Read the model definition and answer for the solid it produces. Units are mm, in the model's axes. A direction names the side the tool comes from. Coordinates: 2 decimals unless noted, no trailing zeros. Write each loop counter-clockwise with the first axis right and the second up, starting at its lowest first coordinate (ties: lowest second). Pieces come first, ordered by that corner, then holes.
1) The part is cut by section C-C (x = -50). Determine the outline of the cut face in (y, z).
2) Each of these flat-tipped pins is pushed along its axis until it touches: pin 1 Ø1 at (y, z) = (-2, 3) entering from +X; pin 2 Ø4 at (x, y) = (-30.5, 26) entering from +Z; pin 3 Ø22.5 at (x, y) = (-50, 0) entering from +Z; pin 4 Ø2 at (x, y) = (-2.5, 16) entering from +Z. Where does it stop, or does it pass through?
3) The part is cut by section D-D (x = -27). Determine the outline of the cut face in (y, z).
4) Find the intervals of material crossed by line 1 (X direction, y = -19, z = 1); line 2 (Y direction, x = -50, z = 9.5); line 3 (Y direction, x = 0, z = 3.1), in increasing order.
5) Which of the six approach directions +Z, -Z, +X, -X, +Y, -Y give full straight-line access (tool end or side, diameter ignored) to faces 1 (the face through (5.2, -1, 3)), 2 (the face through (27.09, 0.37, 8.7)), 3 (the face through (-50.1, 14.4, 8))?
6) The part is cut by section B-B (y = 0). Give the number of separate pieces and of enclosed holes in the cut face, then the cut area to 3 significant figures.
7) The part is cut by section A-A (x = 1.5). Determine the outline of the cut face in (y, z), then the cut area to 3 significant figures.
from build123d import *
from OCP.BRepFilletAPI import BRepFilletAPI_MakeChamfer

# Parameters (mm, degrees)
SKETCH1_R               = 3
SKETCH1_R_2             = 16.15
BOSS_EXTRUDE1_DEPTH     = 12
CUT_EXTRUDE1_DEPTH      = 82.610354735
CUT_EXTRUDE1_DEPTH_BACK = 82.610354735
CUT_EXTRUDE2_DEPTH      = 81.984566431
CUT_EXTRUDE2_DEPTH_BACK = 81.984566431
CUT_EXTRUDE3_DEPTH      = 81.984566431
CUT_EXTRUDE3_DEPTH_BACK = 81.984566431
FILLET1_R               = 1.5
SKETCH5_R               = 18.073165259
SKETCH5_R_2             = 14
BOSS_EXTRUDE2_DEPTH     = 1.5
FILLET2_R               = 5
CHAMFER1_SIZE           = 2
CHAMFER1_SIZE2          = 1.908627476
SKETCH7_R               = 18.5
CUT_EXTRUDE4_DEPTH      = 81.984566431
CHAMFER2_SIZE           = 2
CHAMFER3_SIZE           = 1.5


with BuildPart() as part:
    # Sketch1 → Boss-Extrude1 (new body)
    with BuildSketch(Plane.XY):
        Polygon((-72, 16), (-72, -16), (-55.5, -26), (-16.944232072, -28.942026003), (-8.689847933, -35.598787405), (0, -36.5), (8.689847933, -35.598787405), (16.944232072, -28.942026003), (55.5, -26), (72, -16), (72, 16), (55.5, 26), (16.944232072, 28.942026003), (8.689847933, 35.598787405), (0, 36.5), (-8.689847933, 35.598787405), (-16.944232072, 28.942026003), (-55.5, 26), align=None)
        with Locations((0, 30)):
            Circle(SKETCH1_R, mode=Mode.SUBTRACT)
        with Locations((-50, 0)):
            Circle(SKETCH1_R_2, mode=Mode.SUBTRACT)
        with Locations(Location((0, -30, 0), (0, 0, 180))):
            Circle(SKETCH1_R, mode=Mode.SUBTRACT)
        with Locations(Location((50, 0, 0), (0, 0, 180))):
            Circle(SKETCH1_R_2, mode=Mode.SUBTRACT)
    extrude(amount=BOSS_EXTRUDE1_DEPTH)

    # Sketch2 → Cut-Extrude1 (cut, two sides)
    with BuildSketch(Plane(origin=(0, 0, 0), x_dir=(1, 0, 0), z_dir=(0, 1, 0))) as cut_extrude1_sk:
        Polygon((-31, -12), (-23.3, -5.5), (4.394576276, -5.5), (23.3, -5.5), (31, -12), align=None)
        Polygon((-72, 0), (-72, -6.5), (-37.7, -6.5), (-30, 0), align=None)
        Polygon((30, 0), (72, 0), (72, -6.5), (37.7, -6.5), align=None)
    extrude(amount=CUT_EXTRUDE1_DEPTH, mode=Mode.SUBTRACT)
    extrude(cut_extrude1_sk.sketch, amount=-CUT_EXTRUDE1_DEPTH_BACK, mode=Mode.SUBTRACT)

    # Sketch3 → Cut-Extrude2 (cut, two sides)
    with BuildSketch(Plane.XY.offset(5.5)) as cut_extrude2_sk:
        Polygon((5.2, -10.7), (-5.2, -10.7), (-5.2, 7.758003241), (-2.908652734, 10.7), (2.908652734, 10.7), (5.2, 7.758003241), align=None)
    extrude(amount=CUT_EXTRUDE2_DEPTH, mode=Mode.SUBTRACT)
    extrude(cut_extrude2_sk.sketch, amount=-CUT_EXTRUDE2_DEPTH_BACK, mode=Mode.SUBTRACT)

    # Sketch4 → Cut-Extrude3 (cut, two sides)
    with BuildSketch(Plane.XY.offset(5.5)) as cut_extrude3_sk:
        Polygon((-17, 13.75), (-17, -13.75), (-10.5, -22.5), (-10.5, 22.5), align=None)
        Polygon((17, 13.75), (10.5, 22.5), (10.5, -22.5), (17, -13.75), align=None)
    extrude(amount=CUT_EXTRUDE3_DEPTH, mode=Mode.SUBTRACT)
    extrude(cut_extrude3_sk.sketch, amount=-CUT_EXTRUDE3_DEPTH_BACK, mode=Mode.SUBTRACT)

    # Fillet1
    fillet1_edges = [part.edges().sort_by_distance(p)[0] for p in [
        (-10.5, -22.5, 2.75),
        (-17, -13.75, 2.75),
        (-17, 13.75, 2.75),
        (-10.5, 22.5, 2.75),
        (17, 13.75, 2.75),
        (10.5, -22.5, 2.75),
        (10.5, 22.5, 2.75),
    ]]
    fillet(fillet1_edges, radius=FILLET1_R)

    # Sketch5 → Boss-Extrude2 (add)
    with BuildSketch(Plane.XY.offset(6.5)):
        with Locations((-50, 0)):
            Circle(SKETCH5_R)
        with Locations((-50, 0)):
            Circle(SKETCH5_R_2, mode=Mode.SUBTRACT)
        with Locations((50, 0)):
            Circle(SKETCH5_R)
        with Locations(Location((50, 0, 0), (0, 0, 180))):
            Circle(SKETCH5_R_2, mode=Mode.SUBTRACT)
    extrude(amount=BOSS_EXTRUDE2_DEPTH)

    # Fillet2
    fillet2_edges = [part.edges().sort_by_distance(p)[0] for p in [
        (55.5, 26, 9.25),
        (72, 16, 9.25),
        (72, -16, 9.25),
        (55.5, -26, 9.25),
        (-55.5, -26, 9.25),
        (-72, -16, 9.25),
        (-72, 16, 9.25),
        (-55.5, 26, 9.25),
    ]]
    fillet(fillet2_edges, radius=FILLET2_R)

    # Chamfer1: one chamfer whose edges measure the first distance from different faces: ONE call of the kernel's chamfer builder (chamfer() names one face for all edges)
    chamfer1_edges_1 = [part.edges().sort_by_distance(p)[0] for p in [
        (-27.15, 28.163267435, 8.75),
        (-27.15, -28.163267435, 8.75),
    ]]
    chamfer1_side_1 = [part.faces().sort_by_distance(p)[0] for p in [
        (-27.136613276, 0, 8.738699519),
    ]]
    chamfer1_edges_2 = [part.edges().sort_by_distance(p)[0] for p in [
        (27.15, -28.163267435, 8.75),
        (27.15, 28.163267435, 8.75),
    ]]
    chamfer1_side_2 = [part.faces().sort_by_distance(p)[0] for p in [
        (27.136613276, 0, 8.738699519),
    ]]
    chamfer1_edges_3 = [part.edges().sort_by_distance(p)[0] for p in [
        (-12.817040003, -32.270406704, 5.5),
        (-20.122116036, -28.699535248, 5.5),
        (-20.122116036, 28.699535248, 5.5),
        (-12.817040003, 32.270406704, 5.5),
        (-4.344923967, 36.049393703, 5.5),
        (4.344923967, 36.049393703, 5.5),
        (12.817040003, 32.270406704, 5.5),
        (20.122116036, 28.699535248, 5.5),
        (20.122116036, -28.699535248, 5.5),
        (12.817040003, -32.270406704, 5.5),
        (4.344923967, -36.049393703, 5.5),
        (-4.344923967, -36.049393703, 5.5),
        (42.654881047, 26.980156174, 12),
        (63.056178259, 21.420498025, 12),
        (63.056178259, -21.420498025, 12),
        (72, 0, 12),
        (71.356463181, 15.637521788, 12),
        (71.356463181, -15.637521788, 12),
        (55.457065699, -25.866202879, 12),
        (55.457065699, 25.866202879, 12),
        (-42.654881047, -26.980156174, 12),
        (-63.056178259, -21.420498025, 12),
        (-63.056178259, 21.420498025, 12),
        (-72, 0, 12),
        (-71.356463181, 15.637521788, 12),
        (-71.356463181, -15.637521788, 12),
        (-55.457065699, 25.866202879, 12),
        (-55.457065699, -25.866202879, 12),
        (42.654881047, -26.980156174, 12),
        (-42.654881047, 26.980156174, 12),
    ]]
    chamfer1 = BRepFilletAPI_MakeChamfer(part.part.solid().wrapped)
    for e in chamfer1_edges_1:
        chamfer1.Add(CHAMFER1_SIZE, CHAMFER1_SIZE2, e.wrapped, chamfer1_side_1[0].wrapped)  # the first distance lies on this face
    for e in chamfer1_edges_2:
        chamfer1.Add(CHAMFER1_SIZE, CHAMFER1_SIZE2, e.wrapped, chamfer1_side_2[0].wrapped)  # the first distance lies on this face
    for e in chamfer1_edges_3:
        chamfer1.Add(CHAMFER1_SIZE, e.wrapped)
    add(Compound.cast(chamfer1.Shape()), mode=Mode.REPLACE)

    # Sketch7 → Cut-Extrude4 (cut, through all)
    with BuildSketch(Plane(origin=(0, 0, 6.5), x_dir=(-1, 0, 0), z_dir=(0, 0, -1))):
        with Locations((-50, 0)):
            Circle(SKETCH7_R)
        with Locations((50, 0)):
            Circle(SKETCH7_R)
    extrude(amount=CUT_EXTRUDE4_DEPTH, mode=Mode.SUBTRACT)

    # Chamfer2
    chamfer2_edges = [part.edges().sort_by_distance(p)[0] for p in [
        (17, -0.248090155, 0),
        (14.954115772, 16.504074922, 0),
        (10.5, 0, 0),
        (15.102057886, -16.304922077, 0),
        (-10.5, 0, 0),
        (-14.954115772, -16.504074922, 0),
        (-17, 0, 0),
        (-14.954115772, 16.504074922, 0),
        (16.924109135, 13.724896298, 0),
        (11.528923392, 19.389467286, 0),
        (11.528923392, -19.389467286, 0),
        (-11.528923392, -19.389467286, 0),
        (-16.924109135, -13.724896298, 0),
        (-16.924109135, 13.724896298, 0),
        (-11.528923392, 19.389467286, 0),
    ]]
    chamfer(chamfer2_edges, length=CHAMFER2_SIZE)

    # Chamfer3
    chamfer3_edges = [part.edges().sort_by_distance(p)[0] for p in [
        (15.102057886, -16.304922077, 5.5),
        (14.954115772, 16.504074922, 5.5),
        (17, -0.248090155, 5.5),
        (10.5, 0, 5.5),
        (-10.5, 0, 5.5),
        (-14.954115772, -16.504074922, 5.5),
        (-17, 0, 5.5),
        (-14.954115772, 16.504074922, 5.5),
        (16.924109135, 13.724896298, 5.5),
        (11.528923392, 19.389467286, 5.5),
        (11.528923392, -19.389467286, 5.5),
        (-11.528923392, -19.389467286, 5.5),
        (-16.924109135, -13.724896298, 5.5),
        (-16.924109135, 13.724896298, 5.5),
        (-11.528923392, 19.389467286, 5.5),
    ]]
    chamfer(chamfer3_edges, length=CHAMFER3_SIZE)


solid = part.part
Reported:
1. outline: (-26.42, 6.5) - (-14, 6.5) - (-14, 8) - (-16.15, 8) - (-16.15, 12) - (-24.41, 12) - (-26.42, 10) - close; (14, 6.5) - (26.42, 6.5) - (26.42, 10) - (24.41, 12) - (16.15, 12) - (16.15, 8) - (14, 8) - close
2. pin 1: stops at x = 31.67
2. pin 2: stops at z = 12
2. pin 3: passes through
2. pin 4: stops at z = 5.5
3. outline: (-28.17, 0) - (28.17, 0) - (28.17, 6.13) - (26.17, 8.62) - (-26.17, 8.62) - (-28.17, 6.13) - close
4. line 1: x = -31.18 to -14.35, -9.72 to 9.72, 14.35 to 31.18
4. line 2: y = -26.42 to -16.15, 16.15 to 26.42
4. line 3: y = -36.5 to -33, -27 to -10.7, 10.7 to 27, 33 to 36.5
5. face 1: +Z, -Z
5. face 2: +Z, +Y, -Y
5. face 3: +Z
6. separate pieces: 6
6. enclosed holes: 0
6. area: 359 mm2
7. outline: (-36.34, 0) - (-32.6, 0) - (-32.6, 5.5) - (-34.33, 5.5) - (-36.34, 3.5) - close; (-27.4, 0) - (-10.7, 0) - (-10.7, 5.5) - (-27.4, 5.5) - close; (10.7, 0) - (27.4, 0) - (27.4, 5.5) - (10.7, 5.5) - close; (32.6, 0) - (36.34, 0) - (36.34, 3.5) - (34.33, 5.5) - (32.6, 5.5) - close
7. area: 221 mm2
